Geometry check sheet. Reference: drawing and pictorial views, mm from the part's lowest x, y, z. Round coordinates to 2 decimals unless told otherwise and drop trailing zeros. Write each loop counter-clockwise with the first axis right and the second up, starting at its lowest first coordinate (ties: lowest second). Pieces come first, ordered by that corner, then holes.
Item 1: Depth check by flat-ended pin: pin 1 (3 mm diameter, centred on x = 23, z = 7.5, fed in from +Y). Enter the tip coordinate at first touch or a pass-through.
Item 2: Section check A-A, the plane y = 2. State how many separate pieces and enclosed holes the cut face has, plus the area to 3 significant figures.
Item 3: Material ranges on line 1 along X through (y, z) = (2.5, 7.5); line 2 along Z through (x, y) = (22, 4) (1 decimal); line 3 along Z through (x, y) = (15.5, 1) (1 decimal), recorded low to high.
Item 4: Section check D-D, the plane z = 52. Record the cut outline in (x, y).
Item 5: Release check for a two-part mould opening along Y. For the marked faces 1, 2 and 3 record: pulls with the +Y half, pulls with the -Y half, needs draft (parallel to the pull), parting line crosses it, or undercut.
Item 6: Section check B-B, the plane z = 7.5. Record the cut outline in (x, y).
Item 7: Section check C-C, the plane x = 16. Record the cut outline in (y, z).
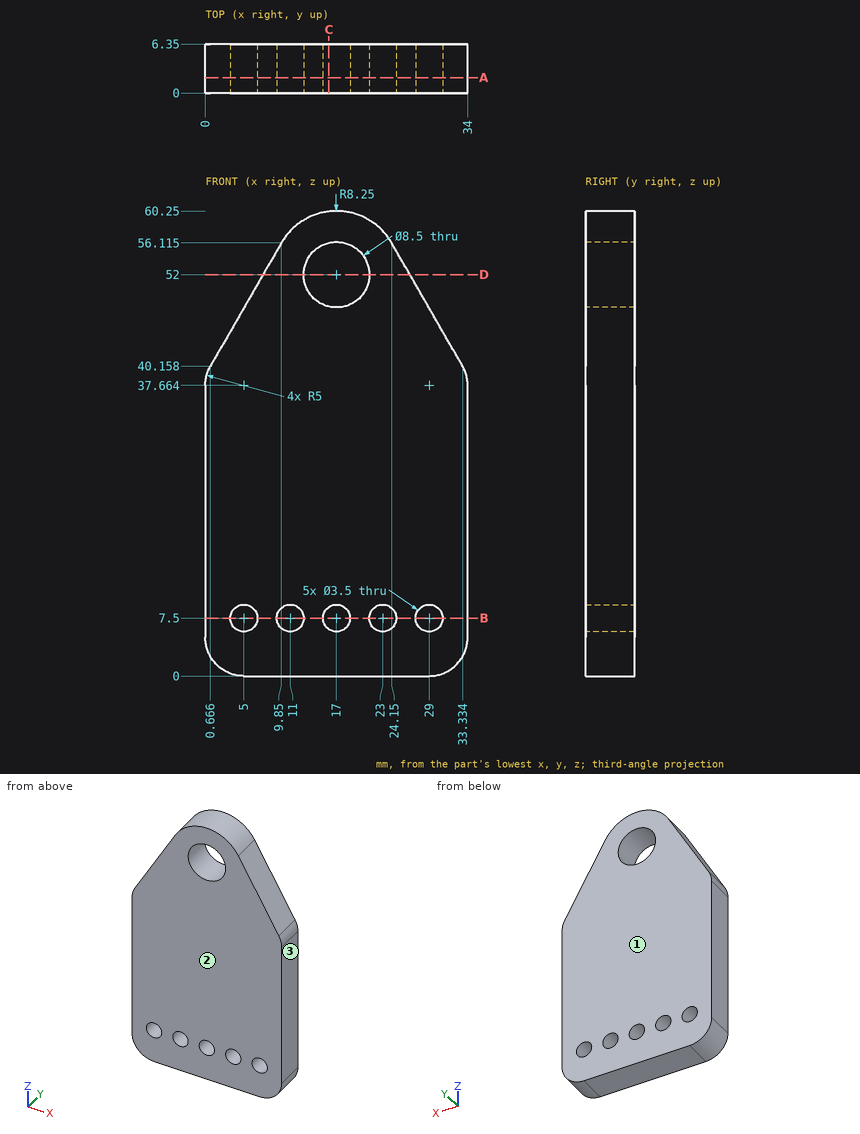
Values found:
1. pin 1: passes through
2. separate pieces: 1
2. enclosed holes: 6
2. area: 1,670 mm2
3. line 1: x = 0 to 3.25, 6.75 to 9.25, 12.75 to 15.25, 18.75 to 21.25, 24.75 to 27.25, 30.75 to 34
3. line 2: z = 0 to 6.1, 8.9 to 58.6
3. line 3: z = 0 to 6.6, 8.4 to 48, 56 to 60.1
4. outline: (7.48, 0) - (12.75, 0) - (12.75, 6.35) - (7.48, 6.35) - close; (21.25, 0) - (26.52, 0) - (26.52, 6.35) - (21.25, 6.35) - close
5. face 1: pulls with the +Y half
5. face 2: pulls with the -Y half
5. face 3: needs draft
6. outline: (0, 0) - (3.25, 0) - (3.25, 6.35) - (0, 6.35) - close; (6.75, 0) - (9.25, 0) - (9.25, 6.35) - (6.75, 6.35) - close; (12.75, 0) - (15.25, 0) - (15.25, 6.35) - (12.75, 6.35) - close; (18.75, 0) - (21.25, 0) - (21.25, 6.35) - (18.75, 6.35) - close; (24.75, 0) - (27.25, 0) - (27.25, 6.35) - (24.75, 6.35) - close; (30.75, 0) - (34, 0) - (34, 6.35) - (30.75, 6.35) - close
7. outline: (0, 0) - (6.35, 0) - (6.35, 6.06) - (0, 6.06) - close; (0, 8.94) - (6.35, 8.94) - (6.35, 47.87) - (0, 47.87) - close; (0, 56.13) - (6.35, 56.13) - (6.35, 60.19) - (0, 60.19) - close
